from build123d import *

# Parameters (mm, degrees)
F0_R           = 12.7
F0_R_2         = 10.3124
F1_DEPTH       = 304.8
F4_D           = 3.9624
F4_DEPTH       = 12.7
F4_CSINK_D     = 5.715
F4_CSINK_ANGLE = 90
F4_TIP         = 1.1904250584
F5_SIZE        = 1.905
F6_SIZE        = 1.905


with BuildPart() as f1:
    # F0 (on Right) → F1 (new body, symmetric)
    with BuildSketch(Plane.YZ):
        Circle(F0_R)
        Circle(F0_R_2, mode=Mode.SUBTRACT)
    extrude(amount=F1_DEPTH, both=True)

    # F4
    with Locations(Plane.XY.offset(12.7)):
        with Locations((-185.7375, 0), (-147.6375, 0), (-109.5375, 0), (-71.4375, 0)):
            CounterSinkHole(F4_D / 2, F4_CSINK_D / 2, depth=F4_DEPTH, counter_sink_angle=F4_CSINK_ANGLE)
            with Locations((0, 0, -(F4_DEPTH + F4_TIP / 2))):  # 118° drill point
                Cone(0, F4_D / 2, F4_TIP, mode=Mode.SUBTRACT)

    # F5
    f5_edges = [f1.edges().sort_by_distance(p)[0] for p in [
        (-304.8, -12.7, 0),
    ]]
    chamfer(f5_edges, length=F5_SIZE)

    # F6
    f6_edges = [f1.edges().sort_by_distance(p)[0] for p in [
        (304.8, -12.7, 0),
    ]]
    chamfer(f6_edges, length=F6_SIZE)


solid = f1.part
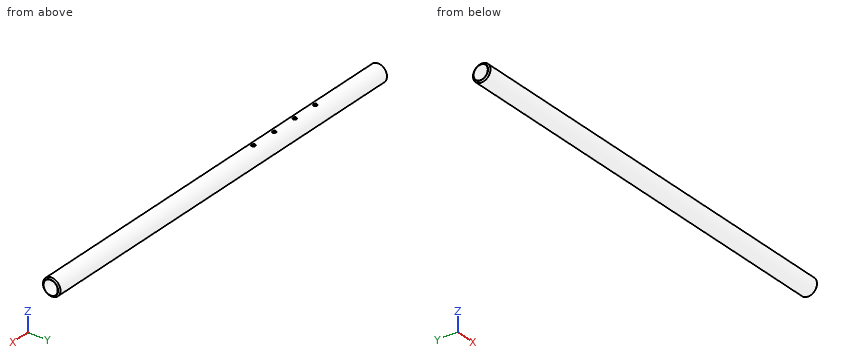
Verification items for the finished model (mm, model axes). Give positions to 0.01 mm unless a question says otherwise; leave off trailing zeros. Order: outer loops, then holes, each group sorted by start corner. A loop starts at its lowest first (then second) coordinate and runs counter-clockwise, first axis right, second up. Notation, with made-up numbers: M 9,-26 L 68,-26 A18 cw 68,-16 Z; hole C 55,1 d9. An arc over 180 degrees is marked long. Answer as a JSON object with one key per item and string values. Group by question number.
1) Depth check by flat-ended pin: pin 1 Ø10 at (x, y) = (223, 9.5) entering from -Z; pin 2 Ø5 at (x, y) = (-71.44, 0) entering from +Z (3 decimals); pin 3 Ø12 at (x, z) = (28.5, -4.5) entering from +Y; pin 4 Ø3 at (x, z) = (85.5, 4) entering from +Y. Enter the tip coordinate at first touch or a pass-through.
2) Cross-section at B-B (x = 55.5). Enter the section's corners in (y, z), then the cut area to 3 significant figures.
3) Scan lines: line 1 along X through (y, z) = (0, 10.8) (3 decimals); line 2 along Y through (x, z) = (-143, -1); line 3 along X through (y, z) = (0, 10.85) (3 decimals). Record each from-to range of solid material in increasing order. Write a range as [from, to].
4) Cross-section at A-A (z = 0). Enter the section's corners in (x, y) (3 decimals).
Result sheet:
{
 "1": {"pin 1": "stops at z = -11.88", "pin 2": "stops at z = 12.345", "pin 3": "stops at y = 12.7", "pin 4": "stops at y = 12.45"},
 "2": {"outline": "C 0,0 d25.4; hole C 0,0 d20.62", "area": "173 mm2"},
 "3": {"line 1": "x = [-304.795, -187.719], [-183.756, -149.619], [-145.656, -111.519], [-107.556, -73.419], [-69.456, 304.795]", "line 2": "y = [-12.66, -10.26], [10.26, 12.66]", "line 3": "x = [-304.745, -187.719], [-183.756, -149.619], [-145.656, -111.519], [-107.556, -73.419], [-69.456, 304.745]"},
 "4": {"outline": "M -304.8,-10.795 L -302.895,-12.7 L 302.895,-12.7 L 304.8,-10.795 L 304.8,-10.312 L -304.8,-10.312 Z; M -304.8,10.312 L 304.8,10.312 L 304.8,10.795 L 302.895,12.7 L -302.895,12.7 L -304.8,10.795 Z"}
}
